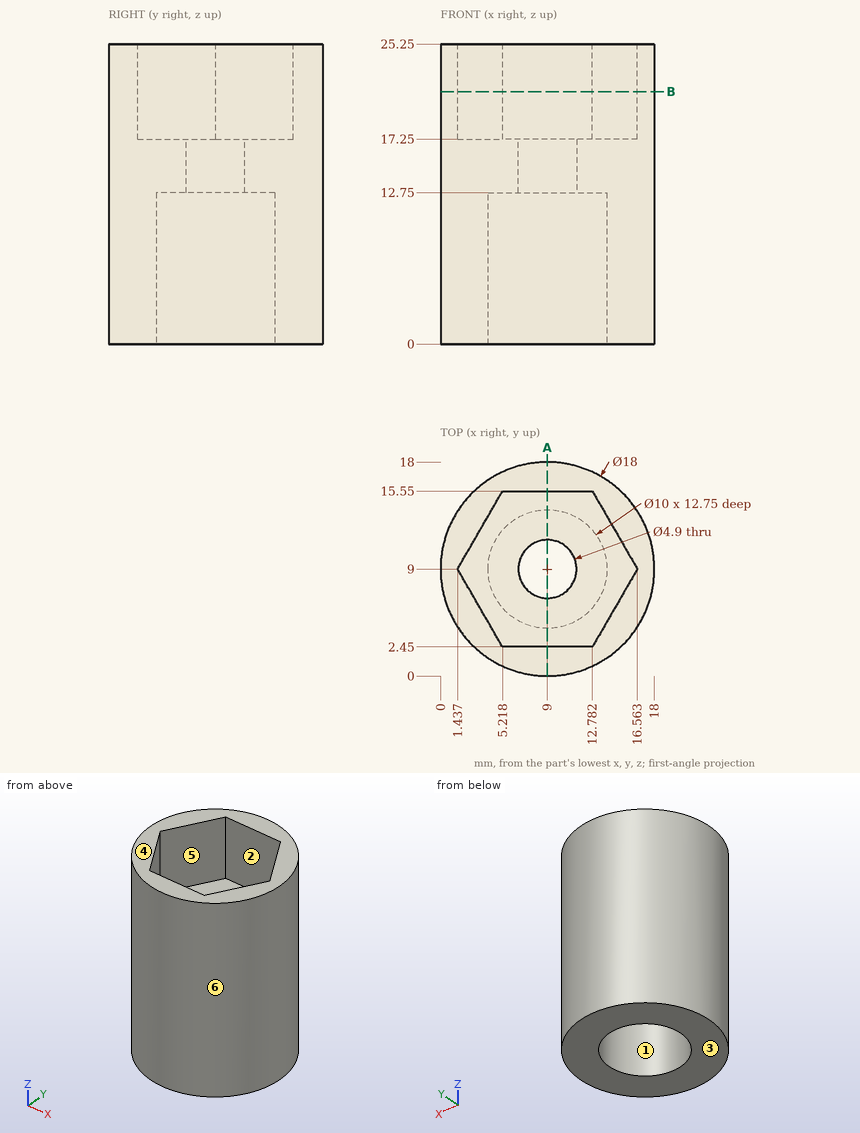
Verification items for this drawing (mm, ordinates from the low corner). A direction names the side the tool comes from. Round coordinates to 2 decimals unless told otherwise and drop trailing zeros. Write each loop counter-clockwise with the first axis right and the second up, starting at its lowest first coordinate (ties: lowest second). Pieces come first, ordered by that corner, then holes. Notation, with made-up numbers: (67, 85.25) - (115, 85.25) arc R21 cw to (115, 92.25) - close; hole circle Ø5 at (2.5, 65.25). An arc over 180 degrees is marked (long way). Answer as a JSON object with one key per item and string values. Group by question number.
Q1. Tool access check on the marked faces 1, 2 and 3. Record the directions out of +Z, -Z, +X, -X, +Y, -Y that give a thin tool (end or side, any length) a straight path to the whole face; none if there is none.
Q2. Mould release check, pull along X, two halves, no side actions. Record for the marked faces 4, 5 and 6: released by +X, released by -X, zero draft, split by the parting line, or undercut.
Q3. Thickness scan on line 1 (Y direction, x = 9, z = 14.55); line 2 (Y direction, x = 9, z = 4.5); line 3 (Z direction, x = 9, y = 13.75). Record the ranges inside material, lowest first.
Q4. Go/stop test with flat-tipped pins: pin 1 Ø2 at (y, z) = (4.5, 7.5) entering from +X; pin 2 Ø9 at (x, y) = (9, 9) entering from -Z; pin 3 Ø5 at (x, y) = (7.5, 11) entering from +Z. Record where each tip stops, or that it passes through.
Q5. Section check A-A, the plane x = 9. Enter the section's corners in (y, z).
Q6. Section check B-B, the plane z = 21.25. Enter the section's corners in (x, y).
Found:
{
 "1": {"face 1": "-Z", "face 2": "+Z", "face 3": "-Z, +X, -X, +Y, -Y"},
 "2": {"face 4": "zero draft", "face 5": "undercut", "face 6": "split by the parting line"},
 "3": {"line 1": "y = 0 to 6.55, 11.45 to 18", "line 2": "y = 0 to 4, 14 to 18", "line 3": "z = 12.75 to 17.25"},
 "4": {"pin 1": "stops at x = 17.29", "pin 2": "stops at z = 12.75", "pin 3": "stops at z = 17.25"},
 "5": {"outline": "(0, 0) - (4, 0) - (4, 12.75) - (6.55, 12.75) - (6.55, 17.25) - (2.45, 17.25) - (2.45, 25.25) - (0, 25.25) - close; (11.45, 12.75) - (14, 12.75) - (14, 0) - (18, 0) - (18, 25.25) - (15.55, 25.25) - (15.55, 17.25) - (11.45, 17.25) - close"},
 "6": {"outline": "circle Ø18 at (9, 9); hole (1.44, 9) - (5.22, 2.45) - (12.78, 2.45) - (16.56, 9) - (12.78, 15.55) - (5.22, 15.55) - close"}
}
